Geometry check sheet. Reference: the model listing, model coordinates, mm. A direction names the side the tool comes from. Coordinates: 2 decimals unless noted, no trailing zeros. Order: outer loops, then holes, each group sorted by start corner. A loop starts at its lowest first (then second) coordinate and runs counter-clockwise, first axis right, second up. Notation, with made-up numbers: M -34,56 L 19,56 A25 ccw 19,88 Z; hole C 28.25,76 d2. An arc over 180 degrees is marked long. One line per item, written item: value. Start each with the question number.
1) Access from +Z, -Z, +X, -X, +Y, -Y to the whole of each face (thin tool, end or side, straight path). Record for faces 5 (the flat face through (2, -5, 0)), 6 (the flat face through (0, 0, 0)), 7 (the flat face through (-40, -10, 9)).
2) Draft check along Z on faces 1 (the flat face through (-21, -11, -21.15)), 2 (the flat face through (-21, -11, 21.15)), 3 (the flat face through (-18, -15, 0)), 4 (the cylindrical face through (0.358, -2.535, 7.823)). Enter one of: pulls with the +Z half, pulls with the -Z half, needs draft (parallel to the pull), parting line crosses it, or undercut.
3) Thickness scan on L1, parallel to X at y = -3.5, z = 10.55; L2, parallel to X at y = -9, z = -7; L3, parallel to Y at x = 6, z = -12. Record the ranges inside material, lowest first. Write a range as from..to.
4) Sectioned sample at A-A, the plane z = -7. Enter the section's corners in (x, y).
5) Go/stop test with flat-tipped pins: P1, Ø17.5, axis at x = -31.15, z = 0, coming from the -Y side; P2, Ø3, axis at y = -4, z = 5.5, coming from the -X side; P3, Ø6.5, axis at x = 0, z = 10.55, coming from the -Y side; P4, Ø8, axis at y = -9.5, z = 8, coming from the +X side. Record where each tip stops, or that it passes through.
6) Sectioned sample at C-C, the plane x = -25. Enter the section's corners in (y, z), then the cut area to 3 significant figures.
7) Sectioned sample at B-B, the plane x = 0. Enter the section's corners in (y, z), then the cut area to 4 significant figures.
8) Sectioned sample at D-D, the plane z = -18. Enter the section's corners in (x, y), then the cut area to 4 significant figures.
```python
from build123d import *

# Parameters (mm, degrees)
F0_W     = 20
F0_H     = 42.3
F1_DEPTH = 5
F2_W     = 5
F2_H     = 42.3
F3_DEPTH = 10
F4_W     = 5
F4_H     = 42.3
F5_DEPTH = 42.3
F6_R     = 11.05
F7_DEPTH = 5.1
F8_D     = 3.3
F9_D     = 5.5


with BuildPart() as f1:
    # F0 (on Front) → F1 (new body)
    with BuildSketch(Plane.XZ):
        Rectangle(F0_W, F0_H)
    extrude(amount=F1_DEPTH)

    # F2 (on face) → F3 (join)
    with BuildSketch(Plane.XZ.offset(5)):
        with Locations((-7.5, 0)):
            Rectangle(F2_W, F2_H)
    extrude(amount=F3_DEPTH)

    # F4 (on face) → F5 (join)
    with BuildSketch(Plane(origin=(-10, 0, 0), x_dir=(0, -1, 0), z_dir=(-1, 0, 0))):
        with Locations((12.5, 0)):
            Rectangle(F4_W, F4_H)
    extrude(amount=F5_DEPTH)

    # F6 (on face) → F7 (cut)
    with BuildSketch(Plane.XZ.offset(15)):
        with Locations((-31.15, 0)):
            Circle(F6_R)
    extrude(amount=-F7_DEPTH, mode=Mode.SUBTRACT)

    # F8 (through all)
    with Locations(Plane.XZ.offset(15)):
        with Locations((-46.6431457505, 15.4931457505), (-15.6568542495, 15.4931457505), (-15.6568542495, -15.4931457505), (-46.6431457505, -15.4931457505)):
            Hole(F8_D / 2)

    # F9 (through all)
    with Locations(Plane(origin=(0, 0, 0), x_dir=(1, 0, 0), z_dir=(0, 1, 0))):
        with Locations((0, -10.55), (0, 10.55)):
            Hole(F9_D / 2)


solid = f1.part
```
Final values:
1. face 5: +Z, -Z, +X, -Y
1. face 6: +Z, -Z, +X, -X, +Y
1. face 7: +Z, -Z, -X, +Y
2. face 1: pulls with the -Z half
2. face 2: pulls with the +Z half
2. face 3: needs draft
2. face 4: undercut
3. L1: x = -10..-2.75, 2.75..10
3. L2: x = -10..-5
3. L3: y = -5..0
4. outline: M -52.3,-15 L -39.7,-15 L -39.7,-10 L -52.3,-10 Z; M -22.6,-15 L -5,-15 L -5,-5 L 10,-5 L 10,0 L -10,0 L -10,-10 L -22.6,-10 Z
5. P1: passes through
5. P2: stops at x = -10
5. P3: stops at y = -5
5. P4: stops at x = -5
6. outline: M -15,-21.15 L -10,-21.15 L -10,-9.18 L -15,-9.18 Z; M -15,9.18 L -10,9.18 L -10,21.15 L -15,21.15 Z
6. area: 120 mm^2
7. outline: M -5,-21.15 L 0,-21.15 L 0,-13.3 L -5,-13.3 Z; M -5,-7.8 L 0,-7.8 L 0,7.8 L -5,7.8 Z; M -5,13.3 L 0,13.3 L 0,21.15 L -5,21.15 Z
7. area: 156.5 mm^2
8. outline: M -52.3,-15 L -5,-15 L -5,-5 L 10,-5 L 10,0 L -10,0 L -10,-10 L -52.3,-10 Z
8. area: 361.5 mm^2
